For this review, take the finished solid that the model builds, in its own axes (mm). A direction names the side the tool comes from. Give positions to 0.01 mm unless a question says otherwise; leave off trailing zeros. Loops run counter-clockwise (first coordinate to the right, second up) from the corner with the lowest first, then second, coordinate; pieces in that order, holes last.
```python
from build123d import *

# Parameters (mm, degrees)
BOSS_EXTRUDE1_DEPTH                        = 609.6
FILLET1_R                                  = 355.6
SKETCH2_R                                  = 31.75
CUT_EXTRUDE1_DEPTH                         = 609.6
SKETCH4_R                                  = 120.65
CUT_EXTRUDE2_DEPTH                         = 88.9
MIRROR1_AT_THE_SECOND_PLANE_COPY_1_SKETC_R = 120.65
MIRROR1_AT_THE_SECOND_PLANE_COPY_1_DEPTH   = 88.9
SHELL1_START                               = 25.4
SHELL1_DEPTH                               = 558.8
SHELL1_START_2                             = 114.3
SHELL1_2_DEPTH                             = 381
BOSS_EXTRUDE6_START                        = -69.85
BOSS_EXTRUDE6_DEPTH                        = 63.5
SKETCH8_R                                  = 19.05
BOSS_EXTRUDE7_DEPTH                        = 63.5
BOSS_EXTRUDE8_START                        = 25.4
SKETCH9_R                                  = 38.1
BOSS_EXTRUDE8_DEPTH                        = 25.4


# Read off the part's stored shape, not the designer's step: Shell1
with BuildPart() as part:
    # Sketch1 → Boss-Extrude1 (new body)
    with BuildSketch(Plane(origin=(0, 0, 0), x_dir=(0, 0, -1), z_dir=(1, 0, 0))):
        Polygon((0, 0), (-406.4, -76.2), (-406.4, 406.4), (-508, 624.281903124), (-508, 914.4), (0, 914.4), align=None)
    extrude(amount=BOSS_EXTRUDE1_DEPTH)

    # Fillet1
    fillet1_edges = [part.edges().sort_by_distance(p)[0] for p in [
        (304.8, 406.4, 406.4),
        (304.8, 624.281903124, 508),
    ]]
    fillet(fillet1_edges, radius=FILLET1_R)

    # Sketch2 → Cut-Extrude1 (cut)
    with BuildSketch(Plane.ZY):
        with Locations((38.1, 228.6)):
            Circle(SKETCH2_R)
        with Locations((38.1, 685.8)):
            Circle(SKETCH2_R)
    extrude(amount=-CUT_EXTRUDE1_DEPTH, mode=Mode.SUBTRACT)

    # Sketch4 → Cut-Extrude2 (cut)
    with BuildSketch(Plane(origin=(609.6, 0, 0), x_dir=(0, 0, -1), z_dir=(1, 0, 0))):
        with Locations((-38.1, 685.8)):
            Circle(SKETCH4_R)
    cut_extrude2 = extrude(amount=-CUT_EXTRUDE2_DEPTH, mode=Mode.SUBTRACT)

    # Mirror1: Cut-Extrude2 across plane
    add(cut_extrude2.mirror(Plane(origin=(304.8, 0, 0), x_dir=(0, 0, 1), z_dir=(1, 0, 0))), mode=Mode.SUBTRACT)

    # Mirror1 at the second plane: Cut-Extrude2 across plane
    add(cut_extrude2.mirror(Plane.ZX.offset(457.2)), mode=Mode.SUBTRACT)

    # Mirror1 at the second plane copy 1 sketc → Mirror1 at the second plane copy 1 (cut)
    with BuildSketch(Plane(origin=(0, 914.4, 0), x_dir=(0, 0, -1), z_dir=(-1, 0, 0))):
        with Locations((-38.1, 685.8)):
            Circle(MIRROR1_AT_THE_SECOND_PLANE_COPY_1_SKETC_R)
    extrude(amount=-MIRROR1_AT_THE_SECOND_PLANE_COPY_1_DEPTH, mode=Mode.SUBTRACT)

    # Shell1 outline → Shell1 (cut)
    with BuildSketch(Plane.YZ.offset(SHELL1_START)):
        with BuildLine():
            Line((374.096778315, 25.4), (540.303221685, 25.4))
            ThreePointArc((540.303221685, 25.4), (685.8, 184.15), (831.296778315, 25.4))
            Line((831.296778315, 25.4), (889, 25.4))
            Line((889, 25.4), (889, 508))
            Line((889, 508), (703.11652516, 508))
            ThreePointArc((703.11652516, 508), (626.150598444, 499.570860132), (552.833471285, 474.68304907))
            Line((552.833471285, 474.68304907), (477.848431839, 439.71695093))
            ThreePointArc((477.848431839, 439.71695093), (404.53130468, 414.829139868), (327.565377964, 406.4))
            Line((327.565377964, 406.4), (-50.357372304, 406.4))
            Line((-50.357372304, 406.4), (21.080127696, 25.4))
            Line((21.080127696, 25.4), (83.103221685, 25.4))
            ThreePointArc((83.103221685, 25.4), (228.6, 184.15), (374.096778315, 25.4))
        make_face()
    extrude(amount=SHELL1_DEPTH, mode=Mode.SUBTRACT)

    # Shell1 2 outline → Shell1 2 (cut)
    with BuildSketch(Plane.YZ.offset(SHELL1_START_2)):
        with BuildLine():
            Line((540.303221685, 25.4), (630.07897614, 25.4))
            ThreePointArc((630.07897614, 25.4), (685.8, 95.25), (741.52102386, 25.4))
            Line((741.52102386, 25.4), (831.296778315, 25.4))
            ThreePointArc((831.296778315, 25.4), (685.8, 184.15), (540.303221685, 25.4))
        make_face()
        with BuildLine():
            Line((284.32102386, 25.4), (374.096778315, 25.4))
            ThreePointArc((374.096778315, 25.4), (228.6, 184.15), (83.103221685, 25.4))
            Line((83.103221685, 25.4), (172.87897614, 25.4))
            ThreePointArc((172.87897614, 25.4), (228.6, 95.25), (284.32102386, 25.4))
        make_face()
    extrude(amount=SHELL1_2_DEPTH, mode=Mode.SUBTRACT)

    # Sketch6 → Boss-Extrude6 (add)
    with BuildSketch(Plane(origin=(0, 0, 0), x_dir=(-1, 0, 0), z_dir=(0, 0, -1)).offset(BOSS_EXTRUDE6_START)):
        with BuildLine():
            Line((-558.8, 914.4), (-514.805909488, 914.4))
            Line((-514.805909488, 914.4), (-337.795567884, 1220.990905122))
            ThreePointArc((-337.795567884, 1220.990905122), (-304.8, 1240.040905122), (-271.804432116, 1220.990905122))
            Line((-271.804432116, 1220.990905122), (-94.794090512, 914.4))
            Line((-94.794090512, 914.4), (-50.8, 914.4))
            Line((-50.8, 914.4), (-271.804432116, 1297.190905122))
            ThreePointArc((-271.804432116, 1297.190905122), (-304.8, 1316.240905122), (-337.795567884, 1297.190905122))
            Line((-337.795567884, 1297.190905122), (-558.8, 914.4))
        make_face()
    extrude(amount=-BOSS_EXTRUDE6_DEPTH)

    # Sketch8 → Boss-Extrude7 (add)
    with BuildSketch(Plane(origin=(0, 0, 69.85), x_dir=(-1, 0, 0), z_dir=(0, 0, -1))):
        with Locations(Location((-304.8, 1278.140905122, 0), (0, 0, 90))):
            Circle(SKETCH8_R)
    extrude(amount=BOSS_EXTRUDE7_DEPTH)

    # Sketch9 → Boss-Extrude8 (add)
    with BuildSketch(Plane(origin=(0, 0, 6.35), x_dir=(-1, 0, 0), z_dir=(0, 0, -1)).offset(BOSS_EXTRUDE8_START)):
        with Locations(Location((-304.8, 1278.140905122, 0), (0, 0, 90))):
            Circle(SKETCH9_R)
    extrude(amount=-BOSS_EXTRUDE8_DEPTH)


solid = part.part
```
Item 1: Take a section at D-D on z = 277.5. Give the boundary of the cut face in (x, y), and give its area (3 significant figures).
Answer:
outline: (0, -52.03) - (609.6, -52.03) - (609.6, 914.4) - (0, 914.4) - close; hole (25.4, -26.19) - (584.2, -26.19) - (584.2, 889) - (25.4, 889) - close
area: 77,700 mm2
Item 2: Take a section at A-A on x = 304.8. Give the boundary of the cut face in (y, z).
Answer:
outline: (-76.2, 406.4) - (0, 0) - (914.4, 0) - (914.4, 508) - (889, 508) - (889, 25.4) - (741.52, 25.4) arc R57.15 ccw (long way) to (630.08, 25.4) - (284.32, 25.4) arc R57.15 ccw (long way) to (172.88, 25.4) - (21.08, 25.4) - (-50.36, 406.4) - close; (1240.04, -19.05) - (1316.24, -19.05) - (1316.24, 6.35) - (1297.19, 6.35) - (1297.19, 69.85) - (1316.24, 69.85) - (1316.24, 133.35) - (1240.04, 133.35) - (1240.04, 69.85) - (1259.09, 69.85) - (1259.09, 6.35) - (1240.04, 6.35) - close; hole circle Ø63.5 at (228.6, 38.1); hole circle Ø63.5 at (685.8, 38.1)
Item 3: Tool access review of faces 5 (the flat face through (301, 464, 0)), 6 (the cylindrical face through (597.078, 403.471, 414.596)), 7 (the flat face through (301, 889, 263)): name each direction out of +Z, -Z, +X, -X, +Y, -Y from which nothing blocks a thin tool from reaching the whole face with its end or side.
Answer:
face 5: -Z, +X, -X, -Y
face 6: +Z, +X, -X, -Y
face 7: +Z
Item 4: Take a section at C-C on x = 242.5. Give the boundary of the cut face in (y, z).
Answer:
outline: (-76.2, 406.4) - (0, 0) - (914.4, 0) - (914.4, 508) - (889, 508) - (889, 25.4) - (741.52, 25.4) arc R57.15 ccw (long way) to (630.08, 25.4) - (284.32, 25.4) arc R57.15 ccw (long way) to (172.88, 25.4) - (21.08, 25.4) - (-50.36, 406.4) - close; (1170.23, 69.85) - (1246.43, 69.85) - (1246.43, 133.35) - (1170.23, 133.35) - close; hole circle Ø63.5 at (228.6, 38.1); hole circle Ø63.5 at (685.8, 38.1)
Item 5: For L1, parallel to X at y = 814.5, z = 274; L2, parallel to Y at x = 337, z = 24.5; L3, parallel to Y at x = 576, z = 38 (3 decimals), list the stretches that pass through material, from the lowest coordinate up.
Answer:
L1: x = 0 to 25.4, 584.2 to 609.6
L2: y = -4.59 to 199.91, 257.29 to 657.11, 714.49 to 914.4
L3: y = -7.125 to 18.718, 82.55 to 107.95, 349.25 to 374.65, 539.75 to 565.15, 806.45 to 831.85, 889 to 914.4
Item 6: Take a section at B-B on y = 228.6. Give the boundary of the cut face in (x, z), and give its area (3 significant figures).
Answer:
outline: (0, 158.75) - (88.9, 158.75) - (88.9, 69.85) - (520.7, 69.85) - (520.7, 158.75) - (609.6, 158.75) - (609.6, 406.4) - (584.2, 406.4) - (584.2, 184.15) - (495.3, 184.15) - (495.3, 95.25) - (114.3, 95.25) - (114.3, 184.15) - (25.4, 184.15) - (25.4, 406.4) - (0, 406.4) - close; (88.9, 0) - (520.7, 0) - (520.7, 6.35) - (88.9, 6.35) - close
area: 34,000 mm2
Item 7: Clearance check with flat-ended pins moving along their axes: pin 1 Ø10 at (x, z) = (243, 275) entering from -Y; pin 2 Ø12 at (x, z) = (357, 268) entering from -Y (3 decimals); pin 3 Ø5 at (x, y) = (225, 410.5) entering from -Z. State where each tip first meets the part, or that it passes through.
Answer:
pin 1: stops at y = -52.5
pin 2: stops at y = -51.375
pin 3: stops at z = 0
Item 8: The part is to be moulded in two halves that separate along Y. For faces 1 (the flat face through (303, -55, 406.4)), 2 (the flat face through (322.3, 1286.1, 6.35)), 3 (the cylindrical face through (43.828, 688.996, 158.708)), 4 (the cylindrical face through (304.241, 1316.237, 101.155)), say which applies: released by +Y, released by -Y, zero draft, split by the parting line, or undercut.
Answer:
face 1: zero draft
face 2: undercut
face 3: undercut
face 4: released by +Y
